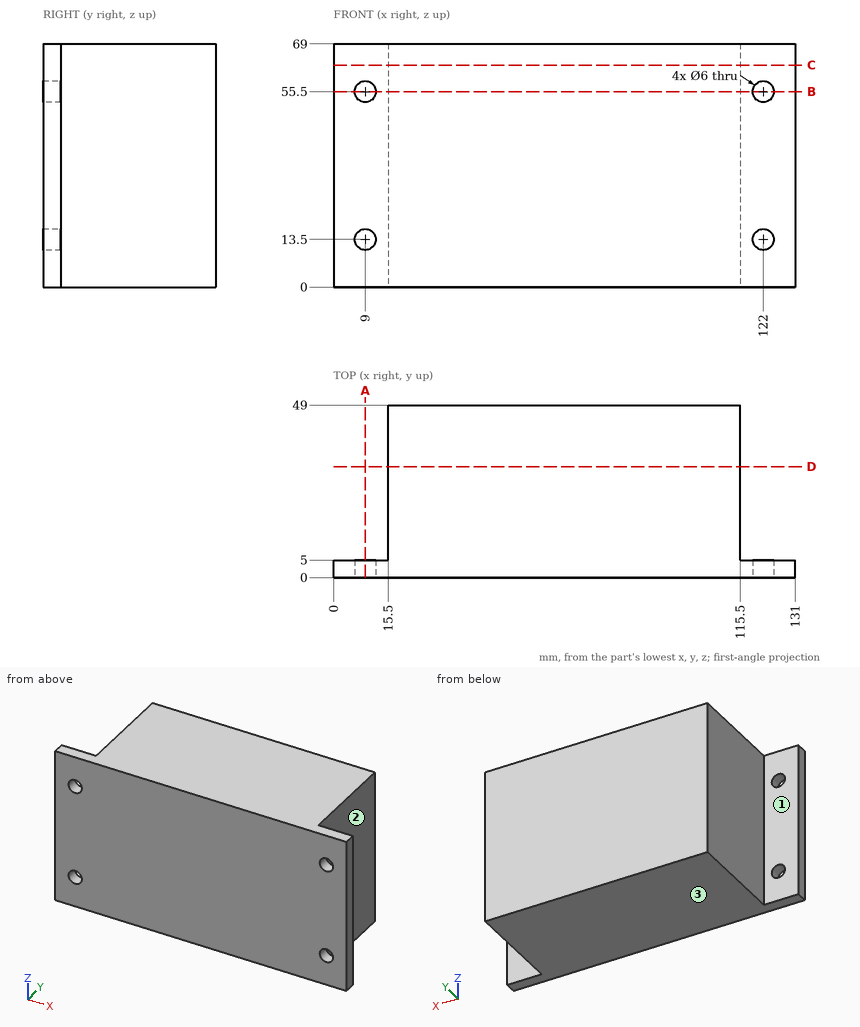
Here's the drawing with two shaded views (mm, measured from the low corner). I have some questions. A direction names the side the tool comes from. Give positions to 0.01 mm unless a question says otherwise; leave off trailing zeros. Loops run counter-clockwise (first coordinate to the right, second up) from the corner with the lowest first, then second, coordinate; pieces in that order, holes last. Notation, with made-up numbers: M 43.25,11 L 93.25,11 A22 cw 93.25,24 Z; hole C 61.25,61 d9. An arc over 180 degrees is marked long. Answer in a Markdown table with one row per item.
1. Suppose I cut it at A-A on x = 9. Write out the boundary of the cut face in (y, z).
Taken from the geometry:
| item | result |
|---|---|
| outline | M 0,0 L 5,0 L 5,10.5 L 0,10.5 Z; M 0,16.5 L 5,16.5 L 5,52.5 L 0,52.5 Z; M 0,58.5 L 5,58.5 L 5,69 L 0,69 Z |
2. Suppose I cut it at D-D on y = 31.5. Write out the boundary of the cut face in (x, z).
Taken from the geometry:
| item | result |
|---|---|
| outline | M 15.5,0 L 115.5,0 L 115.5,69 L 15.5,69 Z |
3. Which directions (+Z, -Z, +X, -X, +Y, -Y) give clear straight access to the entire face, cutting with the end or side of a thin tool? Please do the marked faces 1, 2 and 3.
Taken from the geometry:
| item | result |
|---|---|
| face 1 | +Z, -Z, -X, +Y |
| face 2 | +Z, -Z, +X, +Y |
| face 3 | -Z, +X, -X, +Y, -Y |
4. If I drill on line 1 along X through (y, z) = (3.5, 13.5); line 2 along Y through (x, z) = (119.5, 29); line 3 along X through (y, z) = (30, 37), over which ranges is the centre line in solid material (lowest first)?
Taken from the geometry:
| item | result |
|---|---|
| line 1 | x = 0 to 6, 12 to 119, 125 to 131 |
| line 2 | y = 0 to 5 |
| line 3 | x = 15.5 to 115.5 |
5. Suppose I cut it at C-C on z = 63. Write out the boundary of the cut face in (x, y).
Taken from the geometry:
| item | result |
|---|---|
| outline | M 0,0 L 131,0 L 131,5 L 115.5,5 L 115.5,49 L 15.5,49 L 15.5,5 L 0,5 Z |
6. Suppose I cut it at B-B on z = 55.5. Write out the boundary of the cut face in (x, y), plus the area to 4 significant figures.
Taken from the geometry:
| item | result |
|---|---|
| outline | M 0,0 L 6,0 L 6,5 L 0,5 Z; M 12,0 L 119,0 L 119,5 L 115.5,5 L 115.5,49 L 15.5,49 L 15.5,5 L 12,5 Z; M 125,0 L 131,0 L 131,5 L 125,5 Z |
| area | 4,995 mm² |
7. For pin 1 Ø12 at (x, y) = (46.5, 42) entering from -Z; pin 2 Ø5 at (y, z) = (38.5, 33.5) entering from +X; pin 3 Ø8 at (x, z) = (4, 42) entering from +Y; pin 4 Ø5.5 at (x, z) = (9, 13.5) entering from -Y, each with a flat end and sliding along its axis, tell me the tip position at first contact or that it passes through.
Taken from the geometry:
| item | result |
|---|---|
| pin 1 | stops at z = 0 |
| pin 2 | stops at x = 115.5 |
| pin 3 | stops at y = 5 |
| pin 4 | passes through |
